Could you check a few things on this drawing? It's one solid part, dimensions in mm from its lowest x, y, z. Coordinates: 2 decimals unless noted, no trailing zeros. Order: outer loops, then holes, each group sorted by start corner. A loop starts at its lowest first (then second) coordinate and runs counter-clockwise, first axis right, second up. Notation, with made-up numbers: (22.5, -26.5) - (38.5, -26.5) arc R14 ccw to (38.5, -20.5) - close; hole circle Ø1 at (39.5, 19.25). An arc over 180 degrees is marked (long way). Answer in a Markdown table with one row per item. Add a question column.
Item 1: I want a section at B-B (y = 12). Please give me the cut outline in (x, z) (1 decimal).
Item 2: Will these pins go through, and if not, where does the flat tip stop? pin 1 Ø1.5 at (y, z) = (47, 5.5) entering from +X; pin 2 Ø3 at (x, z) = (182.5, 4) entering from +Y (1 decimal).
Item 3: I want a section at D-D (y = 88.5). Please give me the cut outline in (x, z), plus the area to 3 significant figures.
Item 4: I want a section at A-A (x = 28.5). Please give me the cut outline in (y, z), plus the area to 3 significant figures.
Item 5: If I drill on line 1 along X through (y, z) = (44.5, 0.95) (1 decimal); line 2 along X through (y, z) = (55.5, 2.7) (1 decimal); line 3 along X through (y, z) = (96.5, 4.5) (1 decimal), over which ranges is the centre line in solid material (lowest first)? Write a range as from..to.
Item 6: I want a section at C-C (z = 4.3). Count the separate pieces of the cut face and the enclosed holes in it.
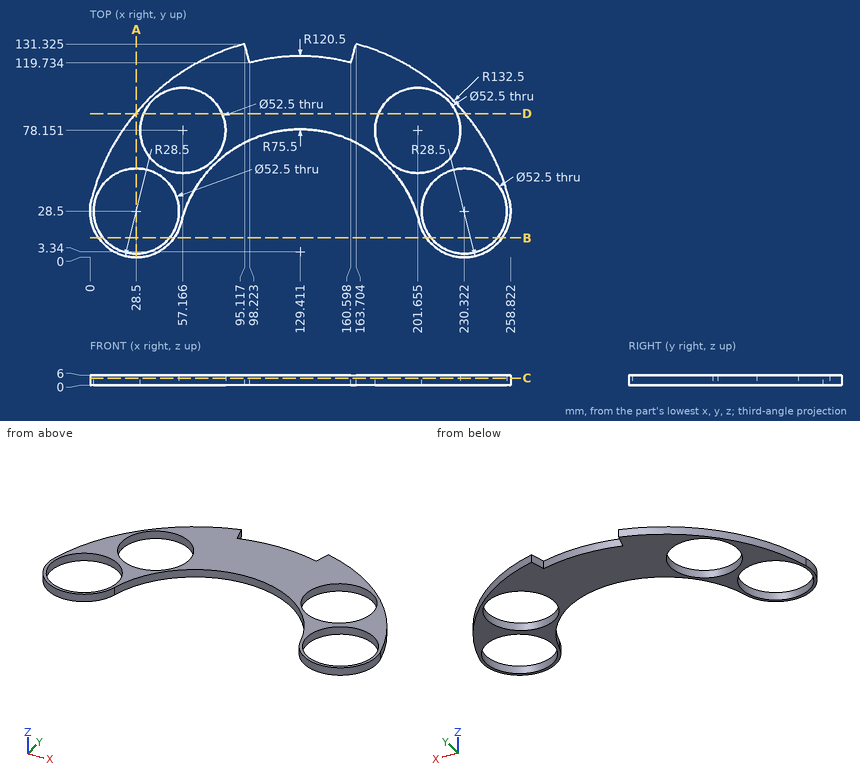
Values follow:
| question | item | result |
|---|---|---|
| 1 | outline | (5.3, 0) - (8.1, 0) - (8.1, 6) - (5.3, 6) - close; (48.9, 0) - (51.7, 0) - (51.7, 6) - (48.9, 6) - close; (207.1, 0) - (209.9, 0) - (209.9, 6) - (207.1, 6) - close; (250.7, 0) - (253.6, 0) - (253.6, 6) - (250.7, 6) - close |
| 2 | pin 1 | stops at x = 254.77 |
| 2 | pin 2 | stops at y = 125.4 |
| 3 | outline | (27.9, 0) - (33.04, 0) - (33.04, 6) - (27.9, 6) - close; (81.29, 0) - (177.53, 0) - (177.53, 6) - (81.29, 6) - close; (225.78, 0) - (230.92, 0) - (230.92, 6) - (225.78, 6) - close |
| 3 | area | 639 mm^2 |
| 4 | outline | (0, 0) - (2.25, 0) - (2.25, 6) - (0, 6) - close; (54.75, 0) - (89.21, 0) - (89.21, 6) - (54.75, 6) - close |
| 4 | area | 220 mm^2 |
| 5 | line 1 | x = 3.5..7.7, 49.3..66.1, 192.7..209.5, 251.1..255.4 |
| 5 | line 2 | x = 7.6..43.9, 70.4..74.8, 184..188.4, 214.9..251.2 |
| 5 | line 3 | x = 35.2..38.4, 75.9..182.9, 220.4..223.6 |
| 6 | separate pieces | 1 |
| 6 | enclosed holes | 4 |
